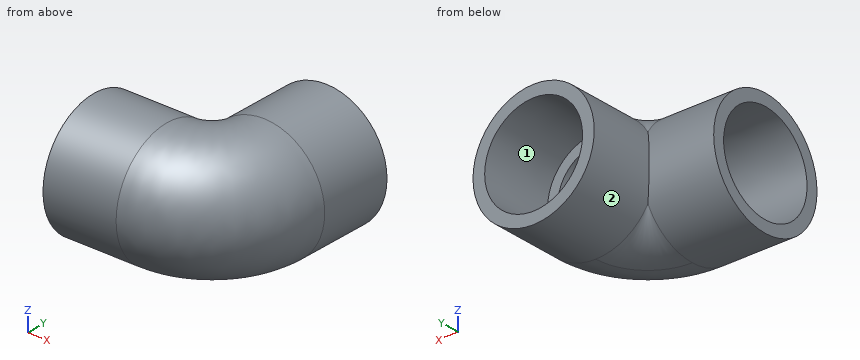
```python
from build123d import *

# Parameters (mm, degrees)
SKETCH3_R   = 16.637
SKETCH3_R_2 = 10.4648


with BuildPart() as part:
    # Sketch1 → Revolve1 (revolve)
    with BuildSketch(Plane.XY):
        Polygon((-34.3408, -16.637), (-14.2748, -16.637), (-14.2748, -13.2842), (-34.3408, -13.4366), align=None)
    revolve(axis=Axis((-34.3408, 0, 0), (1, 0, 0)))



with BuildPart() as body_2:
    # Sketch2 → Revolve2 (revolve)
    with BuildSketch(Plane.XY):
        Polygon((13.4366, 34.3408), (13.2842, 14.2748), (16.637, 14.2748), (16.637, 34.3408), align=None)
    revolve(axis=Axis((0, 0, 0), (0, 1, 0)))


with BuildPart() as part_1:
    add(part.part)

    add(body_2.part)  # Sweep1 merges body 2
    # Sweep1: sweep along a path in Sketch4
    with BuildLine(Plane.XY) as sweep1_path:
        ThreePointArc((-14.2748, 0), (-4.180992, 4.180992), (0, 14.2748))
    # Sketch3 → Sweep1 (sweep)
    with BuildSketch(Plane(origin=(-14.2748, 0, 0), x_dir=(0, 0, -1), z_dir=(1, 0, 0))):
        Circle(SKETCH3_R)
        Circle(SKETCH3_R_2, mode=Mode.SUBTRACT)
    sweep(path=sweep1_path.line)


solid = part_1.part
```
Check sheet for the modelled part. Datum: model origin and axes. Units: mm. Face numbers are marked on the shaded views. Round coordinates to 2 decimals unless told otherwise and drop trailing zeros. Loops run counter-clockwise (first coordinate to the right, second up) from the corner with the lowest first, then second, coordinate; pieces in that order, holes last. Notation, with made-up numbers: (9.5, -8) - (61.5, -8) arc R36 ccw to (61.5, 30) - close; hole circle Ø5 at (7, 82). An arc over 180 degrees is marked (long way). Write item = value, one per line. Start each with the question number.
Q1. Depth check by flat-ended pin: P1, Ø10, axis at x = 4.5, z = -12, coming from the +Y side; P2, Ø2, axis at y = 29, z = -11.5, coming from the +X side (3 decimals); P3, Ø8, axis at x = -22.5, z = 12, coming from the -Y side; P4, Ø6, axis at y = 25, z = 7.5, coming from the -X side. Enter the tip coordinate at first touch or a pass-through.
Q2. Release check for a two-part mould opening along Z. For the marked faces 1 and 2 record: pulls with the +Z half, pulls with the -Z half, needs draft (parallel to the pull), parting line crosses it, or undercut.
Q3. Section check B-B (y = 21). Record the boundary of the cut face in (x, z).
Q4. Section check A-A (y = 28). Record the boundary of the cut face in (x, z).
Q5. Thickness scan on L1, parallel to X at y = 10, z = -6; L2, parallel to Y at x = -22, z = -4; L3, parallel to Z at x = -22, y = -8. Record the ranges inside material, lowest first.
Derived:
q1.P1 = 34.34
q1.P2 = 12.905
q1.P3 = -14.59
q1.P4 = -16.02
q2.face_1 = undercut
q2.face_2 = parting line crosses it
q3.outline = circle Ø33.27 at (0, 0); hole circle Ø26.67 at (0, 0)
q4.outline = circle Ø33.27 at (0, 0); hole circle Ø26.78 at (0, 0)
q5.L1 = -14.27 to -10.5, 8.17 to 15.21
q5.L2 = -16.15 to -12.73, 12.73 to 16.15
q5.L3 = -14.59 to -10.68, 10.68 to 14.59
